Design review of the part built by this model. Coordinates are the model's own, in mm. Face numbers are marked on the shaded views. A direction names the side the tool comes from. Give positions to 0.01 mm unless a question says otherwise; leave off trailing zeros. Order: outer loops, then holes, each group sorted by start corner. A loop starts at its lowest first (then second) coordinate and runs counter-clockwise, first axis right, second up. Notation, with made-up numbers: (-13, -32.75) -> (22, -32.75) arc R17 ccw to (22, -23.75) -> close; hole circle Ø3 at (13, 89.25). An arc over 180 degrees is marked (long way). Use a Markdown table: item, result. Add a question column.
```python
from build123d import *

# Parameters (mm, degrees)
SKETCH1_R             = 32.004
BOSS_EXTRUDE1_DEPTH   = 10.16
SKETCH2_R             = 26.9875
CUT_EXTRUDE1_DEPTH    = 5.08
SKETCH3_R             = 9
CUT_EXTRUDE2_DEPTH    = 4
SKETCH4_R             = 6.5
CUT_EXTRUDE3_DEPTH    = 47.162305315
M4X0_7_TAPPED_HOLE1_D = 3.3


with BuildPart() as part:
    # Sketch1 → Boss-Extrude1 (new body)
    with BuildSketch(Plane.XY):
        Circle(SKETCH1_R)
    extrude(amount=BOSS_EXTRUDE1_DEPTH)

    # Sketch2 → Cut-Extrude1 (cut)
    with BuildSketch(Plane.XY.offset(10.16)):
        Circle(SKETCH2_R)
    extrude(amount=-CUT_EXTRUDE1_DEPTH, mode=Mode.SUBTRACT)

    # Sketch3 → Cut-Extrude2 (cut)
    with BuildSketch(Plane.XY.offset(5.08)):
        Circle(SKETCH3_R)
    extrude(amount=-CUT_EXTRUDE2_DEPTH, mode=Mode.SUBTRACT)

    # Sketch4 → Cut-Extrude3 (cut, through all)
    with BuildSketch(Plane.XY.offset(1.08)):
        Circle(SKETCH4_R)
    extrude(amount=-CUT_EXTRUDE3_DEPTH, mode=Mode.SUBTRACT)

    # M4x0.7 Tapped Hole1 (through all)
    with Locations(Plane.XY.offset(10.16)):
        with Locations((-20.609687798, 20.609687798), (0, 29.1465), (20.609687798, 20.609687798), (29.1465, 0), (20.609687798, -20.609687798), (0, -29.1465), (-20.609687798, -20.609687798), (-29.1465, 0)):
            Hole(M4X0_7_TAPPED_HOLE1_D / 2)


solid = part.part
```
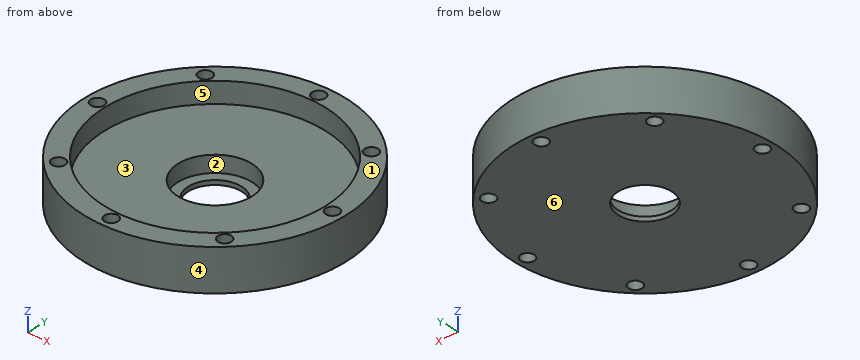
1) Add section A-A (x = 0). Give the boundary of the cut face in (y, z).
2) Machinability: for the marked faces 5 and 6, which of the approach directions +Z, -Z, +X, -X, +Y, -Y give a long, thin tool a straight path to every point of the face, cutting with its end or side? Answer none if there is none.
3) Insertion check: pin 1 (2 mm diameter, centred on x = 22.5, z = 4.5, fed in from +Y); pin 2 (2 mm diameter, centred on y = -24.5, z = 5, fed in from +X); pin 3 (3 mm diameter, centred on x = 23.5, z = 3.5, fed in from +Y); pin 4 (3 mm diameter, centred on x = 0, y = 29.15, fed in from -Z). Each pin has a flat end and moves straight along its axis. Give the tip position at first contact, or say it passes through.
4) For L1, parallel to Y at x = 0, z = 5.5; L2, parallel to X at y = 1, z = 9; L3, parallel to Y at x = 22, z = 9.5, list the stretches that pass through material, from the lowest coordinate up. Write a range as [from, to].
5) Add section C-C (z = 4). Give the number of separate pieces and of enclosed holes in the cut face, then the cut area to 3 significant figures.
6) The part is to be moulded in two halves that separate along Y. For the marked faces 1, 2, 3 and 4, say which applies: +Y half, -Y half, draft (parallel to the pull), parting line (faces both ways), or undercut.
7) Add section D-D (y = 11). Give the boundary of the cut face in (x, z).
Worked answers:
| question | item | result |
|---|---|---|
| 1 | outline | (-32, 0) -> (-30.8, 0) -> (-30.8, 10.16) -> (-32, 10.16) -> close; (-27.5, 0) -> (-6.5, 0) -> (-6.5, 1.08) -> (-9, 1.08) -> (-9, 5.08) -> (-26.99, 5.08) -> (-26.99, 10.16) -> (-27.5, 10.16) -> close; (6.5, 0) -> (27.5, 0) -> (27.5, 10.16) -> (26.99, 10.16) -> (26.99, 5.08) -> (9, 5.08) -> (9, 1.08) -> (6.5, 1.08) -> close; (30.8, 0) -> (32, 0) -> (32, 10.16) -> (30.8, 10.16) -> close |
| 2 | face 5 | +Z |
| 2 | face 6 | -Z, +X, -X, +Y, -Y |
| 3 | pin 1 | y = 23.71 |
| 3 | pin 2 | x = 21.73 |
| 3 | pin 3 | y = 23.24 |
| 3 | pin 4 | through |
| 4 | L1 | [-32, -30.8], [-27.5, -26.99], [26.99, 27.5], [30.8, 32] |
| 4 | L2 | [-31.99, -30.46], [-27.83, -26.97], [26.97, 27.83], [30.46, 31.99] |
| 4 | L3 | [-23.24, -21.5], [-19.72, -15.63], [15.63, 19.72], [21.5, 23.24] |
| 5 | separate pieces | 1 |
| 5 | enclosed holes | 9 |
| 5 | area | 2,890 mm^2 |
| 6 | face 1 | draft |
| 6 | face 2 | undercut |
| 6 | face 3 | undercut |
| 6 | face 4 | parting line |
| 7 | outline | (-30.05, 0) -> (30.05, 0) -> (30.05, 10.16) -> (24.64, 10.16) -> (24.64, 5.08) -> (-24.64, 5.08) -> (-24.64, 10.16) -> (-30.05, 10.16) -> close |
